For this review, take the finished solid that the model builds, in its own axes (mm). Face numbers are marked on the shaded views. A direction names the side the tool comes from. Give positions to 0.01 mm unless a question says otherwise; leave off trailing zeros. Write each loop counter-clockwise with the first axis right and the second up, starting at its lowest first coordinate (ties: lowest second). Pieces come first, ordered by that corner, then holes. Notation, with made-up numbers: (43, 38.25) -> (81, 38.25) arc R28 cw to (81, 62.25) -> close; hole circle Ø2 at (-9, 21.25). An arc over 180 degrees is marked (long way). Write item = value, one per line.
```python
from build123d import *

# Parameters (mm, degrees)
BOSS_EXTRUDE1_DEPTH = 16.5
FILLET1_R           = 1
FILLET2_R           = 1
FILLET3_R           = 1
FILLET4_R           = 1
SKETCH3_R           = 2.85
BOSS_EXTRUDE2_DEPTH = 0.6
SKETCH4_R           = 2.25
BOSS_EXTRUDE3_DEPTH = 7
CUT_EXTRUDE2_DEPTH  = 27.935014386
SKETCH8_R           = 1.75
CUT_EXTRUDE3_DEPTH  = 7


with BuildPart() as part:
    # Sketch1 → Boss-Extrude1 (new body)
    with BuildSketch(Plane(origin=(0, 0, 0), x_dir=(1, 0, 0), z_dir=(0, 1, 0))):
        with BuildLine():
            Line((-0.8, -0.8), (-0.8, -2.102974084))
            ThreePointArc((-0.8, -2.102974084), (0, -2.25), (0.8, -2.102974084))
            Line((0.8, -2.102974084), (0.8, -0.8))
            Line((0.8, -0.8), (2.102974084, -0.8))
            ThreePointArc((2.102974084, -0.8), (2.25, 0), (2.102974084, 0.8))
            Line((2.102974084, 0.8), (0.8, 0.8))
            Line((0.8, 0.8), (0.8, 2.102974084))
            ThreePointArc((0.8, 2.102974084), (0, 2.25), (-0.8, 2.102974084))
            Line((-0.8, 2.102974084), (-0.8, 0.8))
            Line((-0.8, 0.8), (-2.102974084, 0.8))
            ThreePointArc((-2.102974084, 0.8), (-2.25, 0), (-2.102974084, -0.8))
            Line((-2.102974084, -0.8), (-0.8, -0.8))
        make_face()
    extrude(amount=BOSS_EXTRUDE1_DEPTH)

    # Fillet1
    fillet1_edges = [part.edges().sort_by_distance(p)[0] for p in [
        (-2.25, 0, 0),
    ]]
    fillet(fillet1_edges, radius=FILLET1_R)

    # Fillet2
    fillet2_edges = [part.edges().sort_by_distance(p)[0] for p in [
        (0, 0, 2.25),
    ]]
    fillet(fillet2_edges, radius=FILLET2_R)

    # Fillet3
    fillet3_edges = [part.edges().sort_by_distance(p)[0] for p in [
        (2.25, 0, 0),
    ]]
    fillet(fillet3_edges, radius=FILLET3_R)

    # Fillet4
    fillet4_edges = [part.edges().sort_by_distance(p)[0] for p in [
        (0, 0, -2.25),
    ]]
    fillet(fillet4_edges, radius=FILLET4_R)

    # Sketch3 → Boss-Extrude2 (add)
    with BuildSketch(Plane(origin=(0, 16.5, 0), x_dir=(1, 0, 0), z_dir=(0, 1, 0))):
        with Locations(Location((0, 0, 0), (0, 0, 270))):
            Circle(SKETCH3_R)
    extrude(amount=-BOSS_EXTRUDE2_DEPTH)

    # Sketch4 → Boss-Extrude3 (add)
    with BuildSketch(Plane(origin=(0, 16.5, 0), x_dir=(1, 0, 0), z_dir=(0, 1, 0))):
        with Locations(Location((0, 0, 0), (0, 0, 270))):
            Circle(SKETCH4_R)
    extrude(amount=BOSS_EXTRUDE3_DEPTH)

    # Sketch5 → Cut-Extrude2 (cut, through all)
    with BuildSketch(Plane(origin=(10, 0, 0), x_dir=(0, 0, -1), z_dir=(1, 0, 0))):
        with BuildLine():
            Line((-0.5, 21.2), (-0.5, 23.5))
            ThreePointArc((-0.5, 23.5), (0, 24), (0.5, 23.5))
            Line((0.5, 23.5), (0.5, 21.2))
            ThreePointArc((0.5, 21.2), (0, 20.7), (-0.5, 21.2))
        make_face()
    extrude(amount=-CUT_EXTRUDE2_DEPTH, mode=Mode.SUBTRACT)

    # Sketch8 → Cut-Extrude3 (cut)
    with BuildSketch(Plane(origin=(0, 23.5, 0), x_dir=(1, 0, 0), z_dir=(0, 1, 0))):
        with Locations(Location((0, 0, 0), (0, 0, 270))):
            Circle(SKETCH8_R)
    extrude(amount=-CUT_EXTRUDE3_DEPTH, mode=Mode.SUBTRACT)


solid = part.part
```
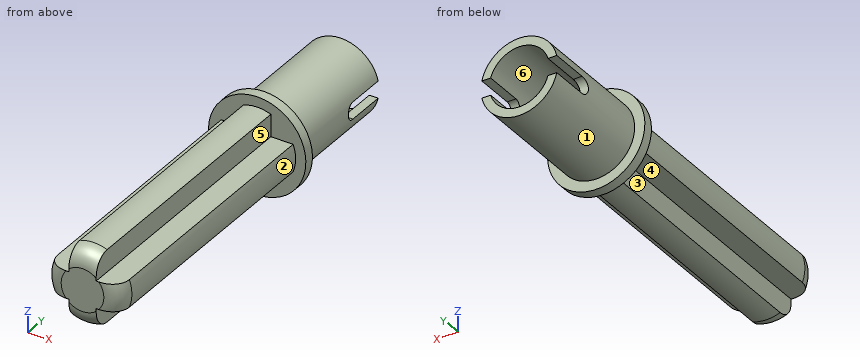
(1) Tool access review of the marked faces 1, 2 and 3: name each direction out of +Z, -Z, +X, -X, +Y, -Y from which nothing blocks a thin tool from reaching the whole face with its end or side.
Answers below:
face_1 = +Y
face_2 = +X, -Y
face_3 = -Z, -X, -Y
(2) Take a section at A-A (x = 0). Write out the cut boundary in (y, z), plus the area to 3 significant figures.
Answers below:
outline = (0, -1.25) arc R1 ccw to (1, -2.25) -> (15.9, -2.25) -> (15.9, -2.85) -> (16.5, -2.85) -> (16.5, -2.25) -> (23.5, -2.25) -> (23.5, -1.75) -> (16.5, -1.75) -> (16.5, 1.75) -> (23.5, 1.75) -> (23.5, 2.25) -> (16.5, 2.25) -> (16.5, 2.85) -> (15.9, 2.85) -> (15.9, 2.25) -> (1, 2.25) arc R1 ccw to (0, 1.25) -> close
area = 81.5 mm^2
(3) Take a section at C-C (z = 0). Write out the cut boundary in (x, y).
Answers below:
outline = (-2.85, 15.9) -> (-2.25, 15.9) -> (-2.25, 1) arc R1 ccw to (-1.25, 0) -> (1.25, 0) arc R1 ccw to (2.25, 1) -> (2.25, 15.9) -> (2.85, 15.9) -> (2.85, 16.5) -> (2.25, 16.5) -> (2.25, 20.7) -> (1.75, 20.7) -> (1.75, 16.5) -> (-1.75, 16.5) -> (-1.75, 20.7) -> (-2.25, 20.7) -> (-2.25, 16.5) -> (-2.85, 16.5) -> close
(4) The part is to be moulded in two halves that separate along X. For the marked faces 4, 5 and 6, say which applies: released by +X, released by -X, zero draft, split by the parting line, or undercut.
Answers below:
face_4 = zero draft
face_5 = released by +X
face_6 = undercut
(5) Take a section at B-B (y = 7.25). Write out the cut boundary in (x, z).
Answers below:
outline = (-2.1, -0.8) -> (-0.8, -0.8) -> (-0.8, -2.1) arc R2.25 ccw to (0.8, -2.1) -> (0.8, -0.8) -> (2.1, -0.8) arc R2.25 ccw to (2.1, 0.8) -> (0.8, 0.8) -> (0.8, 2.1) arc R2.25 ccw to (-0.8, 2.1) -> (-0.8, 0.8) -> (-2.1, 0.8) arc R2.25 ccw to start
(6) To check wall thickness, follow probe 1 along X at (y, z) = (19.25, 0); probe 2 along X at (y, z) = (7.5, 1.2); probe 3 along Y at (x, z) = (0.6, 2.25). State the ranges of each line that lie inside material, in increasing order.
Answers below:
probe_1 = -2.25 to -1.75, 1.75 to 2.25
probe_2 = -0.8 to 0.8
probe_3 = 15.9 to 16.5
(7) For pin 1 (3 mm diameter, centred on y = 7, z = 2, fed in from +X); pin 2 (2 mm diameter, centred on x = 1.5, y = 16, fed in from -Z); pin 3 (0.7 mm diameter, centred on x = 1.5, y = 8, fed in from +Z), all flat-tipped, find the tip position at first contact; note any pin that passes through.
Answers below:
pin_1 = 2.19
pin_2 = -2.81
pin_3 = 0.8
(8) Take a section at D-D (y = 17.75). Write out the cut boundary in (x, z), plus the area to 3 significant figures.
Answers below:
outline = circle Ø4.5 at (0, 0); hole circle Ø3.5 at (0, 0)
area = 6.28 mm^2
